from build123d import *

# Parameters (mm, degrees)
SKETCH1_W           = 35
SKETCH1_H           = 12
SKETCH1_R           = 0.8001
SKETCH1_R_2         = 1.4732
BOSS_EXTRUDE1_DEPTH = 0.2


with BuildPart() as part:
    # Sketch1 → Boss-Extrude1 (new body)
    with BuildSketch(Plane.XY):
        with Locations((17.5, -6)):
            Rectangle(SKETCH1_W, SKETCH1_H)
        with Locations((3.5, -8.3)):
            Circle(SKETCH1_R, mode=Mode.SUBTRACT)
        with Locations((5, -4.5)):
            Circle(SKETCH1_R_2, mode=Mode.SUBTRACT)
        with Locations((30, -4.5)):
            Circle(SKETCH1_R_2, mode=Mode.SUBTRACT)
        with Locations((31.5, -8.3)):
            Circle(SKETCH1_R, mode=Mode.SUBTRACT)
        with BuildLine():
            Line((13.95, -4.5), (13.95, -3.66))
            ThreePointArc((13.95, -3.66), (14.067157288, -3.377157288), (14.35, -3.26))
            Line((14.35, -3.26), (20.65, -3.26))
            ThreePointArc((20.65, -3.26), (20.932842712, -3.377157288), (21.05, -3.66))
            Line((21.05, -3.66), (21.05, -4.5))
            ThreePointArc((21.05, -4.5), (20.576794919, -4.744948974), (20.65, -4.217157288))
            Line((20.65, -4.217157288), (20.65, -4.06))
            ThreePointArc((20.65, -4.06), (20.562132034, -3.847867966), (20.35, -3.76))
            Line((20.35, -3.76), (14.65, -3.76))
            ThreePointArc((14.65, -3.76), (14.437867966, -3.847867966), (14.35, -4.06))
            Line((14.35, -4.06), (14.35, -4.217157288))
            ThreePointArc((14.35, -4.217157288), (14.423205081, -4.744948974), (13.95, -4.5))
        make_face(mode=Mode.SUBTRACT)
        with BuildLine():
            Line((14.35, -2.11), (14.35, -1.782842712))
            ThreePointArc((14.35, -1.782842712), (14.423205081, -1.255051026), (13.95, -1.5))
            Line((13.95, -1.5), (13.95, -2.61))
            ThreePointArc((13.95, -2.61), (14.037867966, -2.822132034), (14.25, -2.91))
            Line((14.25, -2.91), (20.75, -2.91))
            ThreePointArc((20.75, -2.91), (20.962132034, -2.822132034), (21.05, -2.61))
            Line((21.05, -2.61), (21.05, -1.5))
            ThreePointArc((21.05, -1.5), (20.576794919, -1.255051026), (20.65, -1.782842712))
            Line((20.65, -1.782842712), (20.65, -2.11))
            ThreePointArc((20.65, -2.11), (20.562132034, -2.322132034), (20.35, -2.41))
            Line((20.35, -2.41), (14.65, -2.41))
            ThreePointArc((14.65, -2.41), (14.437867966, -2.322132034), (14.35, -2.11))
        make_face(mode=Mode.SUBTRACT)
    extrude(amount=BOSS_EXTRUDE1_DEPTH)


solid = part.part
Could you check a few things on this model? Use its own coordinates, in mm. Give positions to 0.01 mm unless a question says otherwise; leave off trailing zeros. Order: outer loops, then holes, each group sorted by start corner. A loop starts at its lowest first (then second) coordinate and runs counter-clockwise, first axis right, second up.
1. Will this pin go through, and if not, where does the flat tip stop? P1, Ø1, axis at x = 31.5, y = -8.3, coming from the -Z side.
2. I need wall thicknesses on L1, parallel to Y at x = 17.5, z = 0.1; L2, parallel to X at y = -1.5, z = 0.15; L3, parallel to X at y = -2.5, z = 0.05. Which ranges of each line are inside material? Lowest first, please.
3. Suppose I cut it at D-D (z = 0.1). Give the number of separate pieces and of enclosed holes in the cut face, plus the area to 3 significant figures.
4. Suppose I cut it at A-A (y = -8.3). List the corners of the cut face in (x, z) for me, plus the area to 3 significant figures.
5. Suppose I cut it at C-C (x = 30). List the corners of the cut face in (y, z) for me, plus the area to 3 significant figures.
6. Suppose I cut it at B-B (x = 16). List the corners of the cut face in (y, z) for me, plus the area to 3 significant figures.
Solved:
1. P1: passes through
2. L1: y = -12 to -3.76, -3.26 to -2.91, -2.41 to 0
2. L2: x = 0 to 13.95, 14.55 to 20.45, 21.05 to 35
2. L3: x = 0 to 13.95, 21.05 to 35
3. separate pieces: 1
3. enclosed holes: 6
3. area: 393 mm2
4. outline: (0, 0) - (2.7, 0) - (2.7, 0.2) - (0, 0.2) - close; (4.3, 0) - (30.7, 0) - (30.7, 0.2) - (4.3, 0.2) - close; (32.3, 0) - (35, 0) - (35, 0.2) - (32.3, 0.2) - close
4. area: 6.36 mm2
5. outline: (-12, 0) - (-5.97, 0) - (-5.97, 0.2) - (-12, 0.2) - close; (-3.03, 0) - (0, 0) - (0, 0.2) - (-3.03, 0.2) - close
5. area: 1.81 mm2
6. outline: (-12, 0) - (-3.76, 0) - (-3.76, 0.2) - (-12, 0.2) - close; (-3.26, 0) - (-2.91, 0) - (-2.91, 0.2) - (-3.26, 0.2) - close; (-2.41, 0) - (0, 0) - (0, 0.2) - (-2.41, 0.2) - close
6. area: 2.20 mm2
